For this review, use the dimensioned drawing (mm, ordinates from the lowest corner) and the shaded views. Coordinates: 2 decimals unless noted, no trailing zeros. Write each loop counter-clockwise with the first axis right and the second up, starting at its lowest first coordinate (ties: lowest second). Pieces come first, ordered by that corner, then holes. Notation, with made-up numbers: (39.25, -17.5) - (82.25, -17.5) arc R14 ccw to (82.25, 5.5) - close; hole circle Ø10 at (27.25, 70.25). An arc over 180 degrees is marked (long way). One line per item, written item: value.
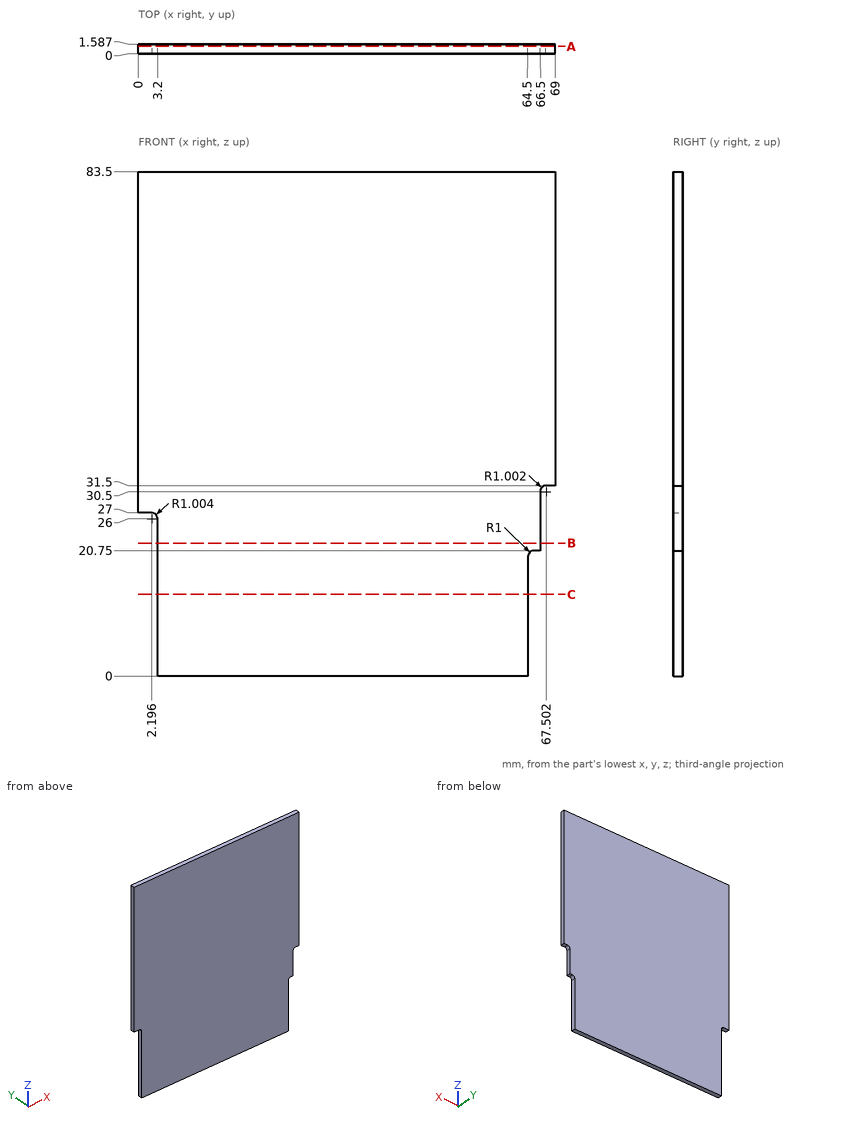
1. Consider section B-B, the plane z = 22. Write out the cut boundary in (x, y).
Answer block:
outline: (3.2, 0) - (66.5, 0) - (66.5, 1.59) - (3.2, 1.59) - close
2. Insertion check: pin 1 Ø0.8 at (y, z) = (1, 24) entering from +X; pin 2 Ø0.5 at (x, y) = (68.5, 0.5) entering from -Z; pin 3 Ø0.5 at (x, y) = (1, 0.5) entering from -Z. Each pin has a flat end and moves straight along its axis. Give the tip position at first contact, or say it passes through.
Answer block:
pin 1: stops at x = 66.5
pin 2: stops at z = 31.5
pin 3: stops at z = 27
3. Consider section C-C, the plane z = 13.5. Write out the cut boundary in (x, y).
Answer block:
outline: (3.2, 0) - (64.5, 0) - (64.5, 1.59) - (3.2, 1.59) - close
4. Consider section A-A, the plane y = 1.2. Write out the cut boundary in (x, z).
Answer block:
outline: (0, 27) - (2.28, 27) arc R1 cw to (3.2, 26) - (3.2, 0) - (64.5, 0) - (64.5, 19.75) arc R1 cw to (65.5, 20.75) - (66.5, 20.75) - (66.5, 30.5) arc R1 cw to (67.44, 31.5) - (69, 31.5) - (69, 83.5) - (0, 83.5) - close
5. Wall thickness on line 1 along X through (y, z) = (0.55, 24); line 2 along X through (y, z) = (1.5, 28.5): over which ranges is each line inside the solid? List them lowest first.
Answer block:
line 1: x = 3.2 to 66.5
line 2: x = 0 to 66.5
